```python
from build123d import *

# Parameters (mm, degrees)
F1_DEPTH = 5.08


with BuildPart() as f1:
    # F0 (on Front) → F1 (new body)
    with BuildSketch(Plane.XZ):
        Polygon((143.185273, -21.642312), (143.185273, 1.702374), (122.968182, -9.969969), (102.751091, 1.702374), (102.751091, -21.642312), (82.534, -33.314655), (102.751091, -44.986997), (102.751091, -68.331683), (122.968182, -56.65934), (143.185273, -68.331683), (143.185273, -44.986997), (163.402364, -33.314655), align=None)
        Polygon((111.641093, -50.119643), (114.07818, -51.526695), (111.641093, -52.933748), align=None, mode=Mode.SUBTRACT)
        Polygon((134.295271, -52.933748), (131.858184, -51.526695), (134.295271, -50.119643), align=None, mode=Mode.SUBTRACT)
        Polygon((102.751091, -31.907602), (102.751091, -34.721707), (100.314004, -33.314655), align=None, mode=Mode.SUBTRACT)
        Polygon((122.968182, -46.39405), (111.641093, -39.854352), (111.641093, -26.774957), (122.968182, -20.235259), (134.295271, -26.774957), (134.295271, -39.854352), align=None, mode=Mode.SUBTRACT)
        Polygon((114.07818, -15.102614), (111.641093, -16.509667), (111.641093, -13.695561), align=None, mode=Mode.SUBTRACT)
        Polygon((143.185273, -34.721707), (143.185273, -31.907602), (145.62236, -33.314655), align=None, mode=Mode.SUBTRACT)
        Polygon((134.295271, -16.509667), (131.858184, -15.102614), (134.295271, -13.695561), align=None, mode=Mode.SUBTRACT)
    extrude(amount=F1_DEPTH)


solid = f1.part
```
Work out the finished part from the listing and answer in its coordinate system (mm). A direction names the side the tool comes from. Give positions to 0.01 mm unless a question says otherwise; leave off trailing zeros. Loops run counter-clockwise (first coordinate to the right, second up) from the corner with the lowest first, then second, coordinate; pieces in that order, holes last. Notation, with made-up numbers: (-25, -30.5) -> (-21, -30.5) arc R20 ccw to (-21, -26.5) -> close; hole circle Ø8 at (15, 70.5). An arc over 180 degrees is marked (long way). Write item = value, one per line. Start each with the question number.
(1) Find section A-A on z = -5.5. Give the vertices of the cut face in (x, y), and give its area (3 significant figures).
(2) Find section C-C on x = 113. Give the vertices of the cut face in (y, z).
(3) Find section D-D on y = -3.2. Give the number of separate pieces and of enclosed holes in the cut face, and give its area (3 significant figures).
(4) Which of the six approach directions +Z, -Z, +X, -X, +Y, -Y give full straight-line access (tool end or side, diameter ignored) to faces 4 (the flat face through (153.152, -2.504, -39.233)), 5 (the flat face through (102.751, -3, -10)), 6 (the flat face through (111.641, -3, -33)), 7 (the flat face through (102.751, -3, -56))?
(5) Find section B-B on x = 127. Give the vertices of the cut face in (y, z), and give its area (3 significant figures).
(6) The mould has two halves that part along Z. Classify faces 1 (the flat face through (112.877, -2.504, -15.796)), 2 (the flat face through (92.5, -2.5, -39.07)), 3 (the flat face through (113, 0, -25)): +Z half, -Z half, draft (parallel to the pull), parting line (faces both ways), or undercut.
(7) Given pin 1 Ø2 at (y, z) = (-2.5, -60) entering from +X; pin 2 Ø1.5 at (x, y) = (106.5, -3) entering from +Z; pin 3 Ø2.5 at (y, z) = (-3, -15.5) entering from -X, each flat-ended and moving along its own axis, determine where each tip first touches the part or whether it passes through.
(8) Find the intervals of material crossed by probe 1 along X at (y, z) = (-2.1, -14.5); probe 2 along X at (y, z) = (-3.7, -46.5); probe 3 along X at (y, z) = (-1.3, -35.5), in increasing order. Write a range as from..to.
From the geometry:
q1.outline = (102.75, -5.08) -> (115.23, -5.08) -> (115.23, 0) -> (102.75, 0) -> close; (130.71, -5.08) -> (143.19, -5.08) -> (143.19, 0) -> (130.71, 0) -> close
q1.area = 127 mm^2
q2.outline = (-5.08, -62.41) -> (0, -62.41) -> (0, -52.15) -> (-5.08, -52.15) -> close; (-5.08, -50.9) -> (0, -50.9) -> (0, -40.64) -> (-5.08, -40.64) -> close; (-5.08, -25.99) -> (0, -25.99) -> (0, -15.73) -> (-5.08, -15.73) -> close; (-5.08, -14.48) -> (0, -14.48) -> (0, -4.21) -> (-5.08, -4.21) -> close
q3.separate_pieces = 1
q3.enclosed_holes = 7
q3.area = 2,370 mm^2
q4.face_4 = -Z, +X, +Y, -Y
q4.face_5 = +Z, -X, +Y, -Y
q4.face_6 = +Y, -Y
q4.face_7 = -Z, -X, +Y, -Y
q5.outline = (-5.08, -58.99) -> (0, -58.99) -> (0, -44.07) -> (-5.08, -44.07) -> close; (-5.08, -22.56) -> (0, -22.56) -> (0, -7.64) -> (-5.08, -7.64) -> close
q5.area = 152 mm^2
q6.face_1 = undercut
q6.face_2 = -Z half
q6.face_3 = draft
q7.pin_1 = 143.19
q7.pin_2 = -0.03
q7.pin_3 = 102.75
q8.probe_1 = 102.75..111.64, 113.03..132.9, 134.3..143.19
q8.probe_2 = 102.75..143.19
q8.probe_3 = 86.32..111.64, 134.3..159.62
